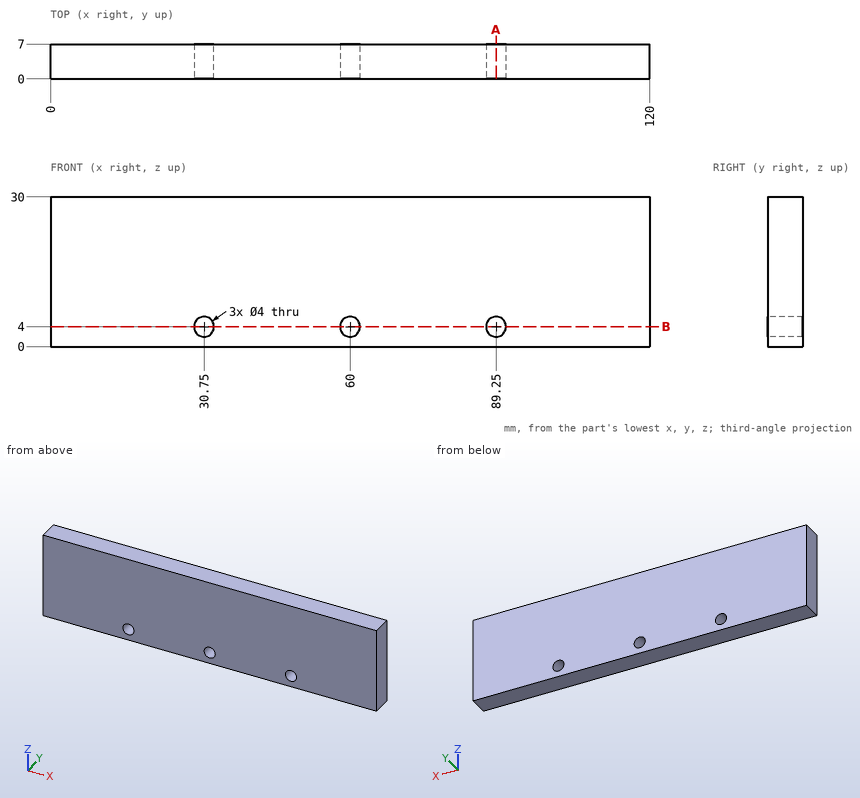
Answer from the drawing. Dimensions are ordinates in mm from the lowest x, y and z of the part. Round coordinates to 2 decimals unless told otherwise and drop trailing zeros. Write each loop counter-clockwise with the first axis right and the second up, starting at its lowest first coordinate (ties: lowest second). Pieces come first, ordered by that corner, then holes. Notation, with made-up numbers: M 23,38 L 49,38 A35 ccw 49,71 Z; hole C 71,-25.5 d8. An arc over 180 degrees is marked long. One line per item, written item: value.
Q1. A straight line is drawn through the part: line 1 (Z direction, x = 30.75, y = 4). Find the intervals that lie inside material, in ascending order. Write a range as [from, to].
Data:
line 1: [0, 2], [6, 30]
Q2. Find section B-B on z = 4. Write down the section's boundary in (x, y), plus the area to 3 significant figures.
Data:
outline: M 0,0 L 28.75,0 L 28.75,7 L 0,7 Z; M 32.75,0 L 58,0 L 58,7 L 32.75,7 Z; M 62,0 L 87.25,0 L 87.25,7 L 62,7 Z; M 91.25,0 L 120,0 L 120,7 L 91.25,7 Z
area: 756 mm2
Q3. Find section A-A on x = 89.25. Write down the section's boundary in (y, z), plus the area to 3 significant figures.
Data:
outline: M 0,0 L 7,0 L 7,2 L 0,2 Z; M 0,6 L 7,6 L 7,30 L 0,30 Z
area: 182 mm2
